Verification items for the finished model (mm, model axes). A direction names the side the tool comes from. Coordinates: 2 decimals unless noted, no trailing zeros. Write each loop counter-clockwise with the first axis right and the second up, starting at its lowest first coordinate (ties: lowest second). Pieces come first, ordered by that corner, then holes. Notation, with made-up numbers: M 83.5,82.25 L 142.5,82.25 A8 cw 142.5,96.25 Z; hole C 25,-32.75 d1. An arc over 180 degrees is marked long. One line per item, written item: value.
```python
from build123d import *

# Parameters (mm, degrees)
SKETCH1_W           = 15
SKETCH1_H           = 15
BOSS_EXTRUDE1_DEPTH = 15
SKETCH2_W           = 2.69425289
SKETCH2_H           = 15
CUT_EXTRUDE1_DEPTH  = 10
SKETCH3_R           = 2.15
CUT_EXTRUDE2_DEPTH  = 37


with BuildPart() as part:
    # Sketch1 → Boss-Extrude1 (new body)
    with BuildSketch(Plane.XY):
        Rectangle(SKETCH1_W, SKETCH1_H)
    extrude(amount=BOSS_EXTRUDE1_DEPTH)

    # Sketch2 → Cut-Extrude1 (cut)
    with BuildSketch(Plane.ZY.offset(7.5)):
        with Locations((7.5, 0)):
            Rectangle(SKETCH2_W, SKETCH2_H)
    extrude(amount=-CUT_EXTRUDE1_DEPTH, mode=Mode.SUBTRACT)

    # Sketch3 → Cut-Extrude2 (cut)
    with BuildSketch(Plane.XY.offset(15)):
        with Locations((-2.5, 0)):
            Circle(SKETCH3_R)
    extrude(amount=-CUT_EXTRUDE2_DEPTH, mode=Mode.SUBTRACT)


solid = part.part
```
Item 1: Cross-section at D-D, the plane y = -4. Enter the section's corners in (x, z).
The answers:
outline: M -7.5,0 L 7.5,0 L 7.5,15 L -7.5,15 L -7.5,8.85 L 2.5,8.85 L 2.5,6.15 L -7.5,6.15 Z
Item 2: Scan lines: line 1 (Z direction, x = -4.25, y = -6.25); line 2 (Y direction, x = -2.5, z = 12.75); line 3 (Y direction, x = -3.5, z = 12). Record each from-to range of solid material in increasing order.
The answers:
line 1: z = 0 to 6.15, 8.85 to 15
line 2: y = -7.5 to -2.15, 2.15 to 7.5
line 3: y = -7.5 to -1.9, 1.9 to 7.5
Item 3: Cross-section at A-A, the plane x = 1. Enter the section's corners in (y, z).
The answers:
outline: M -7.5,0 L 7.5,0 L 7.5,6.15 L -7.5,6.15 Z; M -7.5,8.85 L 7.5,8.85 L 7.5,15 L -7.5,15 Z
Item 4: Access from +Z, -Z, +X, -X, +Y, -Y to the whole of each face (thin tool, end or side, straight path). Record for faces 1 (the face through (0, 0, 0)), 2 (the face through (2.5, 0, 7)).
The answers:
face 1: -Z, +X, -X, +Y, -Y
face 2: -X, +Y, -Y
Item 5: Cross-section at B-B, the plane y = 0. Enter the section's corners in (x, z).
The answers:
outline: M -7.5,0 L -4.65,0 L -4.65,6.15 L -7.5,6.15 Z; M -7.5,8.85 L -4.65,8.85 L -4.65,15 L -7.5,15 Z; M -0.35,0 L 7.5,0 L 7.5,15 L -0.35,15 L -0.35,8.85 L 2.5,8.85 L 2.5,6.15 L -0.35,6.15 Z
Item 6: Go/stop test with flat-tipped pins: P1, Ø1.3, axis at y = -3.5, z = 8, coming from the -X side; P2, Ø3.5, axis at x = -2.5, y = 0, coming from the -Z side. Record where each tip stops, or that it passes through.
The answers:
P1: stops at x = 2.5
P2: passes through
Item 7: Draft check along X on faces 3 (the face through (-5, 0, 8.847)), 4 (the face through (-4.206, -1.308, 3.12)), 5 (the face through (-7.5, 0, 3)). Enter one of: released by +X, released by -X, zero draft, split by the parting line, or undercut.
The answers:
face 3: zero draft
face 4: undercut
face 5: released by -X
Item 8: Cross-section at C-C, the plane x = -2.5. Enter the section's corners in (y, z), and give its area (3 significant figures).
The answers:
outline: M -7.5,0 L -2.15,0 L -2.15,6.15 L -7.5,6.15 Z; M -7.5,8.85 L -2.15,8.85 L -2.15,15 L -7.5,15 Z; M 2.15,0 L 7.5,0 L 7.5,6.15 L 2.15,6.15 Z; M 2.15,8.85 L 7.5,8.85 L 7.5,15 L 2.15,15 Z
area: 132 mm²
